Can you work these out from the model? Positions are in its coordinate system, mm. A direction names the side the tool comes from. Coordinates: 2 decimals unless noted, no trailing zeros. Order: outer loops, then holes, each group sorted by start corner. A loop starts at its lowest first (then second) coordinate and runs counter-clockwise, first axis right, second up. Notation, with made-up numbers: (18, 59.5) -> (36, 59.5) arc R14 cw to (36, 68.5) -> close; hole circle Ø11 at (27.5, -18). An arc over 180 degrees is marked (long way). Use a Markdown table: item, result. Add a question column.
1. Suppose I cut it at A-A, the plane x = 0. List the corners of the cut face in (y, z) for me, then the cut area to 3 significant figures.
2. For pin 1 Ø9 at (x, y) = (-86.92, 31.64) entering from -Z (3 decimals); pin 2 Ø1 at (y, z) = (35.5, 10) entering from +X; pin 3 Ø10 at (x, z) = (52.5, 5.5) entering from +Y; pin 4 Ø4 at (y, z) = (27, 2.5) entering from +X, each with a flat end and sliding along its axis, tell me the tip position at first contact or that it passes through.
3. If I drill on line 1 along X through (y, z) = (-30.5, 6.5); line 2 along X through (y, z) = (-1, 14); line 3 along Z through (x, y) = (45.5, -89.5), over which ranges is the centre line in solid material (lowest first)? Write a range as from..to.
4. Suppose I cut it at B-B, the plane y = 0. List the corners of the cut face in (x, z) for me.
5. Suppose I cut it at D-D, the plane x = 93. List the corners of the cut face in (y, z) for me.
6. We'd pull the mould along Y, two halves only. Please class faces 3 (the flat face through (52, 2, 0)), 4 (the cylindrical face through (97.119, -1.915, 8.112)), 5 (the cylindrical face through (-16.8, -75.657, 18.788)): pulls with the +Y half, pulls with the -Y half, needs draft (parallel to the pull), parting line crosses it, or undercut.
7. Suppose I cut it at C-C, the plane z = 12.75. State how many separate pieces and enclosed holes the cut face has, then the cut area to 3 significant figures.
8. For faces 1 (the flat face through (-2, -78, 16)), 2 (the cylindrical face through (-43.94, -84.54, 8.11)), which set-ups out of +Z, -Z, +X, -X, +Y, -Y let a thin tool reach every point of the face, with its end or its side?
```python
from build123d import *

# Parameters (mm, degrees)
SKETCH1_R           = 120
BOSS_EXTRUDE1_DEPTH = 21.5
SKETCH2_OUTSIDE_W   = 310.018
SKETCH2_OUTSIDE_H   = 310.018
SKETCH2_OUTSIDE_R   = 77.5
CUT_EXTRUDE1_DEPTH  = 5.5
SKETCH3_R           = 5
CUT_EXTRUDE2_DEPTH  = 171.458206021
CIRPATTERN1_COUNT   = 9
SKETCH4_R           = 50
CUT_EXTRUDE3_DEPTH  = 172.062123218


with BuildPart() as part:
    # Sketch1 → Boss-Extrude1 (new body)
    with BuildSketch(Plane.XY):
        Circle(SKETCH1_R)
    extrude(amount=BOSS_EXTRUDE1_DEPTH)

    # Sketch2 outside → Cut-Extrude1 (cut)
    with BuildSketch(Plane.XY.offset(21.5)):
        Rectangle(SKETCH2_OUTSIDE_W, SKETCH2_OUTSIDE_H)
        Circle(SKETCH2_OUTSIDE_R, mode=Mode.SUBTRACT)
    extrude(amount=-CUT_EXTRUDE1_DEPTH, mode=Mode.SUBTRACT)

    # Sketch3 → Cut-Extrude2 (cut, through all)
    with BuildSketch(Plane.XY.offset(16)):
        with Locations((92.5, 0)):
            Circle(SKETCH3_R)
    cut_extrude2 = extrude(amount=-CUT_EXTRUDE2_DEPTH, mode=Mode.SUBTRACT)

    # CirPattern1: Cut-Extrude2 ×9 about axis
    cirpattern1_axis = Axis((0, 0, 0), (0, 0, 1))
    for i in range(1, CIRPATTERN1_COUNT):
        add(cut_extrude2.rotate(cirpattern1_axis, i * 360 / CIRPATTERN1_COUNT), mode=Mode.SUBTRACT)

    # Sketch4 → Cut-Extrude3 (cut, through all)
    with BuildSketch(Plane.XY.offset(21.5)):
        Circle(SKETCH4_R)
    extrude(amount=-CUT_EXTRUDE3_DEPTH, mode=Mode.SUBTRACT)


solid = part.part
```
Worked out:
| question | item | result |
|---|---|---|
| 1 | outline | (-120, 0) -> (-50, 0) -> (-50, 21.5) -> (-77.5, 21.5) -> (-77.5, 16) -> (-120, 16) -> close; (50, 0) -> (120, 0) -> (120, 16) -> (77.5, 16) -> (77.5, 21.5) -> (50, 21.5) -> close |
| 1 | area | 2,540 mm² |
| 2 | pin 1 | passes through |
| 2 | pin 2 | stops at x = 114.78 |
| 2 | pin 3 | stops at y = 110.2 |
| 2 | pin 4 | stops at x = 117.37 |
| 3 | line 1 | x = -116.06..-91.79, -82.05..-39.62, 39.62..116.06 |
| 3 | line 2 | x = -120..-49.99, 49.99..87.6, 97.4..120 |
| 3 | line 3 | z = 0..16 |
| 4 | outline | (-120, 0) -> (-50, 0) -> (-50, 21.5) -> (-77.5, 21.5) -> (-77.5, 16) -> (-120, 16) -> close; (50, 0) -> (87.5, 0) -> (87.5, 16) -> (77.5, 16) -> (77.5, 21.5) -> (50, 21.5) -> close; (97.5, 0) -> (120, 0) -> (120, 16) -> (97.5, 16) -> close |
| 5 | outline | (-75.84, 0) -> (-4.97, 0) -> (-4.97, 16) -> (-75.84, 16) -> close; (4.97, 0) -> (75.84, 0) -> (75.84, 16) -> (4.97, 16) -> close |
| 6 | face 3 | needs draft |
| 6 | face 4 | undercut |
| 6 | face 5 | parting line crosses it |
| 7 | separate pieces | 1 |
| 7 | enclosed holes | 10 |
| 7 | area | 36,700 mm² |
| 8 | face 1 | +Z |
| 8 | face 2 | +Z, -Z |
